Geometry check sheet. Reference: the model listing, model coordinates, mm. A direction names the side the tool comes from. Round coordinates to 2 decimals unless told otherwise and drop trailing zeros. Order: outer loops, then holes, each group sorted by start corner. A loop starts at its lowest first (then second) coordinate and runs counter-clockwise, first axis right, second up.
Autodesk Inventor part; units mm, degrees
ref_plane "YZ Plane" through (0, 0, 0) normal (1, 0, 0) x (0, 1, 0)
ref_plane "XZ Plane" through (0, 0, 0) normal (0, 1, 0) x (-1, 0, 0)
ref_plane "XY Plane" through (0, 0, 0) normal (0, 0, 1) x (1, 0, 0)
sketch "Sketch1" plane through (0, 0, 0) normal (0, 0, 1) x (1, 0, 0)
  circle A0 centre (-53.0097, 46.3835) radius 44.45
  point P0 (0, 0)
  dimension "d0" = 88.9
extrude "Extrusion1" add sketch "Sketch1" along normal blind 584.2
sketch "Sketch2" plane through (-53.0097, 46.3835, 0) normal (0, 0, -1) x (-1, 0, 0)
  circle A0 centre (0, 0) radius 44.45
  circle A1 centre (0, 0) radius 50.5264
  point P0 (-53.0097, -46.3835)
  dimension "d3" = 6.0764
extrude "Extrusion2" add sketch "Sketch2" against normal blind 50.8 contours A0 | A1
sketch "Sketch3" plane through (-53.0097, 46.3835, 584.2) normal (0, 0, 1) x (1, 0, 0)
  circle A0 centre (0, 0) radius 44.45
  circle A1 centre (0, 0) radius 38.354
  point P0 (53.0097, -46.3835)
  dimension "d6" = 6.096
extrude "Extrusion3" cut sketch "Sketch3" against normal blind 581.025 contours A1
sketch "Sketch4" plane through (-53.0097, 46.3835, 0) normal (0, 0, -1) x (-1, 0, 0)
  circle A0 centre (0, 0) radius 16.637
  point P0 (-53.0097, -46.3835)
  dimension "d9" = 33.274
extrude "Extrusion4" add sketch "Sketch4" along normal blind 38.1
thread "Thread1"
properties part number "long pipe"
(1) Sectioned sample at D-D, the plane x = -81. Record the cut outline in (y, z) (3 decimals), and give its area (3 significant figures).
Returned:
outline: (4.319, 0) - (88.448, 0) - (88.448, 50.8) - (80.914, 50.8) - (80.914, 584.2) - (72.605, 584.2) - (72.605, 3.175) - (20.162, 3.175) - (20.162, 584.2) - (11.853, 584.2) - (11.853, 50.8) - (4.319, 50.8) - close
area: 10,600 mm2
(2) Depth check by flat-ended pin: P1, Ø3, axis at y = 38, z = 457, coming from the -X side; P2, Ø23, axis at x = -41, y = 62.5, coming from the +Z side (3 decimals); P3, Ø1.5, axis at x = -87.5, z = 182.5, coming from the -Y side. Enter the tip coordinate at first touch or a pass-through.
Returned:
P1: stops at x = -96.92
P2: stops at z = 3.175
P3: stops at y = 17.45
(3) Set-up check for faces 1 (the flat face through (-52.8, 1.7, 50.8)), 2 (the flat face through (-64.9, 58.3, 0)), 3 (the cylindrical face through (-46.43, 96.48, 25.04)): record each of +Z, -Z, +X, -X, +Y, -Y from which the full face is reachable in a straight line by a thin tool's end or side.
Returned:
face 1: +Z
face 2: -Z
face 3: +Z, -Z
(4) Sectioned sample at B-B, the plane y = 52. Record the cut outline in (x, z) (3 decimals), and give its area (3 significant figures).
Returned:
outline: (-103.223, 0) - (-68.67, 0) - (-68.67, -38.1) - (-37.349, -38.1) - (-37.349, 0) - (-2.796, 0) - (-2.796, 50.8) - (-8.916, 50.8) - (-8.916, 584.2) - (-15.069, 584.2) - (-15.069, 3.175) - (-90.95, 3.175) - (-90.95, 584.2) - (-97.103, 584.2) - (-97.103, 50.8) - (-103.223, 50.8) - close
area: 9,250 mm2
(5) Sectioned sample at A-A, the plane x = -58. Record the cut outline in (y, z) (3 decimals).
Returned:
outline: (-3.896, 0) - (30.513, 0) - (30.513, -38.1) - (62.254, -38.1) - (62.254, 0) - (96.663, 0) - (96.663, 50.8) - (90.552, 50.8) - (90.552, 584.2) - (84.411, 584.2) - (84.411, 3.175) - (8.356, 3.175) - (8.356, 584.2) - (2.215, 584.2) - (2.215, 50.8) - (-3.896, 50.8) - close
(6) Sectioned sample at C-C, the plane z = 538. Record the cut outline in (x, y), and give its area (3 significant figures).
Returned:
outline: circle Ø88.9 at (-53.01, 46.38); hole circle Ø76.71 at (-53.01, 46.38)
area: 1,590 mm2
(7) Draft check along X on faces 4 (the flat face through (-89.4, 33.4, 584.2)), 5 (the cylindrical face through (-85.77, 16.34, 313.77)), 6 (the cylindrical face through (-91.327, 48.07, 297.755)), 7 (the flat face through (-54, 47, 3.175)). Enter one of: released by +X, released by -X, zero draft, split by the parting line, or undercut.
Returned:
face 4: zero draft
face 5: split by the parting line
face 6: undercut
face 7: undercut
(8) Material ranges on line 1 (X direction, y = 49, z = 105); line 2 (X direction, y = 46.5, z = 208); line 3 (Y direction, x = -54.5, z = 215.5), recorded low to high.
Returned:
line 1: x = -97.38 to -91.27, -14.75 to -8.64
line 2: x = -97.46 to -91.36, -14.66 to -8.56
line 3: y = 1.96 to 8.06, 84.71 to 90.81
